Can you work these out from the drawing? Everything is in mm from the part's minimum corner. Round coordinates to 2 decimals unless told otherwise and drop trailing zeros. Write each loop counter-clockwise with the first axis right and the second up, starting at its lowest first coordinate (ties: lowest second). Pieces come first, ordered by that corner, then holes. Notation, with made-up numbers: (-35, 7.5) - (18, 7.5) arc R25 ccw to (18, 23.5) - close; hole circle Ø6 at (-39.75, 42.5). An arc over 180 degrees is marked (long way). One line per item, written item: value. Start each with the question number.
Item 1: If I drill on line 1 (Y direction, x = 14.5, z = 5); line 2 (X direction, y = 14, z = 27.5); line 3 (X direction, y = 8, z = 4.5), over which ranges is the centre line in solid material (lowest first)?
Item 2: Thinking about a two-plate mould opening in Y: for the marked faces 1 and 2, which applies, released by +Y, released by -Y, zero draft, split by the parting line, or undercut?
Item 3: Imagine slicing it at C-C, the plane z = 27.5. Please give me the cut outline in (x, y).
Item 4: For P1, Ø5.5, axis at x = 96, z = 4.5, coming from the +Y side; P2, Ø10, axis at y = 24.5, z = 9, coming from the +X side; P3, Ø10, axis at x = 88, y = 20.5, coming from the +Z side; P4, Ø12, axis at x = 74, y = 21.5, coming from the -Z side, each with a flat end and sliding along its axis, tell me the tip position at first contact or that it passes through.
Item 5: Imagine slicing it at B-B, the plane y = 23. Please give me the cut outline in (x, z).
Item 6: Imagine slicing it at D-D, the plane x = 14.5. Please give me the cut outline in (y, z).
Item 7: Imagine slicing it at A-A, the plane x = 164.5. Please give me the cut outline in (y, z).
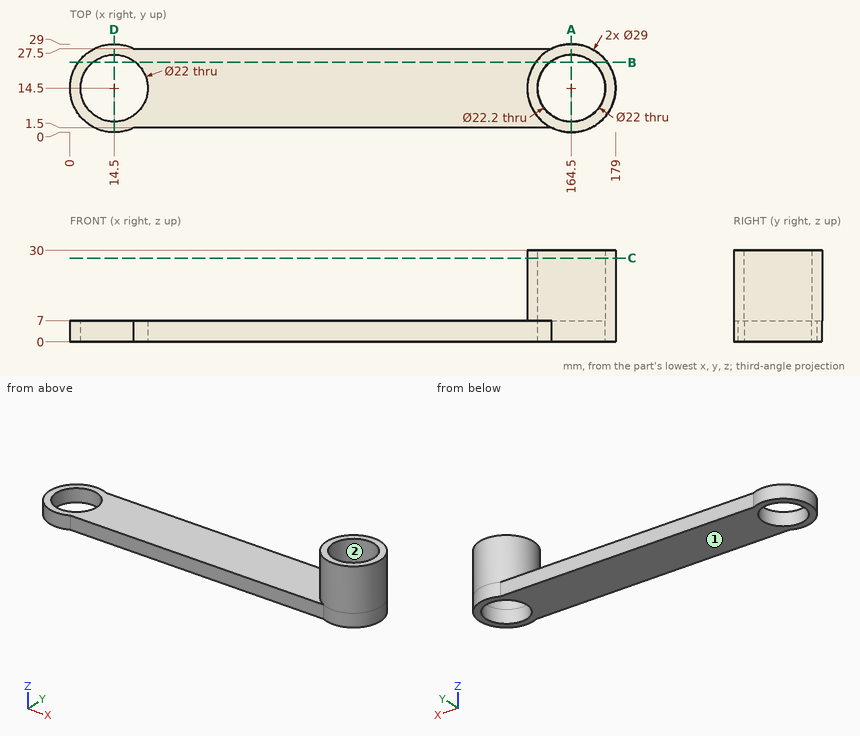
Values follow:
1. line 1: y = 0 to 3.5, 25.5 to 29
1. line 2: x = 150.01 to 153.41, 175.59 to 178.99
1. line 3: x = 1.54 to 5.63, 23.37 to 155.63, 173.37 to 177.46
2. face 1: zero draft
2. face 2: undercut
3. outline: circle Ø29 at (164.5, 14.5); hole circle Ø22.2 at (164.5, 14.5)
4. P1: stops at y = 27.5
4. P2: stops at x = 178.11
4. P3: stops at z = 7
4. P4: stops at z = 0
5. outline: (2.75, 0) - (7.52, 0) - (7.52, 7) - (2.75, 7) - close; (21.48, 0) - (157.52, 0) - (157.52, 7) - (157.36, 7) - (157.36, 30) - (152.75, 30) - (152.75, 7) - (21.48, 7) - close; (171.48, 0) - (176.25, 0) - (176.25, 30) - (171.64, 30) - (171.64, 7) - (171.48, 7) - close
6. outline: (0, 0) - (3.5, 0) - (3.5, 7) - (0, 7) - close; (25.5, 0) - (29, 0) - (29, 7) - (25.5, 7) - close
7. outline: (0, 0) - (3.5, 0) - (3.5, 7) - (3.4, 7) - (3.4, 30) - (0, 30) - close; (25.5, 0) - (29, 0) - (29, 30) - (25.6, 30) - (25.6, 7) - (25.5, 7) - close
